Input: dimensioned drawing with shaded views. Units: mm. Origin: part minimum x, y, z. Give positions to 0.01 mm unless a question says otherwise; leave off trailing zeros. Loops run counter-clockwise (first coordinate to the right, second up) from the corner with the lowest first, then second, coordinate; pieces in that order, holes last. Notation, with made-up numbers: M 54,-4 L 103,-4 A14 cw 103,6 Z; hole C 44.5,-26 d1. An arc over 180 degrees is marked long. Use CSV: the item, a comma, the result in double quotes. Start each with the question number.
Q1. Pin query (flat end, axial travel): pin 1 (2 mm diameter, centred on x = 2.5, z = 53.5, fed in from -Y) (1 decimal); pin 2 (1 mm diameter, centred on x = 3, y = 63, fed in from +Z); pin 3 (1.5 mm diameter, centred on x = 1, y = 137, fed in from -Z). Return the tip coordinate at first contact, or that it passes through.
Q2. Section A-A, the plane x = 1.5. Output: boundary loops of the cut face in (y, z) (1 decimal), plus the area to 3 significant figures.
Q3. Section C-C, the plane z = 10. Output: boundary loops of the cut face in (x, y).
Q4. Material intervals for line 1 along Y through (x, z) = (4.75, 50) (1 decimal); line 2 along Z through (x, y) = (4, 18) (1 decimal); line 3 along Z through (x, y) = (1.5, 126), sorted ascending.
Q5. Section B-B, the plane y = 112. Output: boundary loops of the cut face in (x, z).
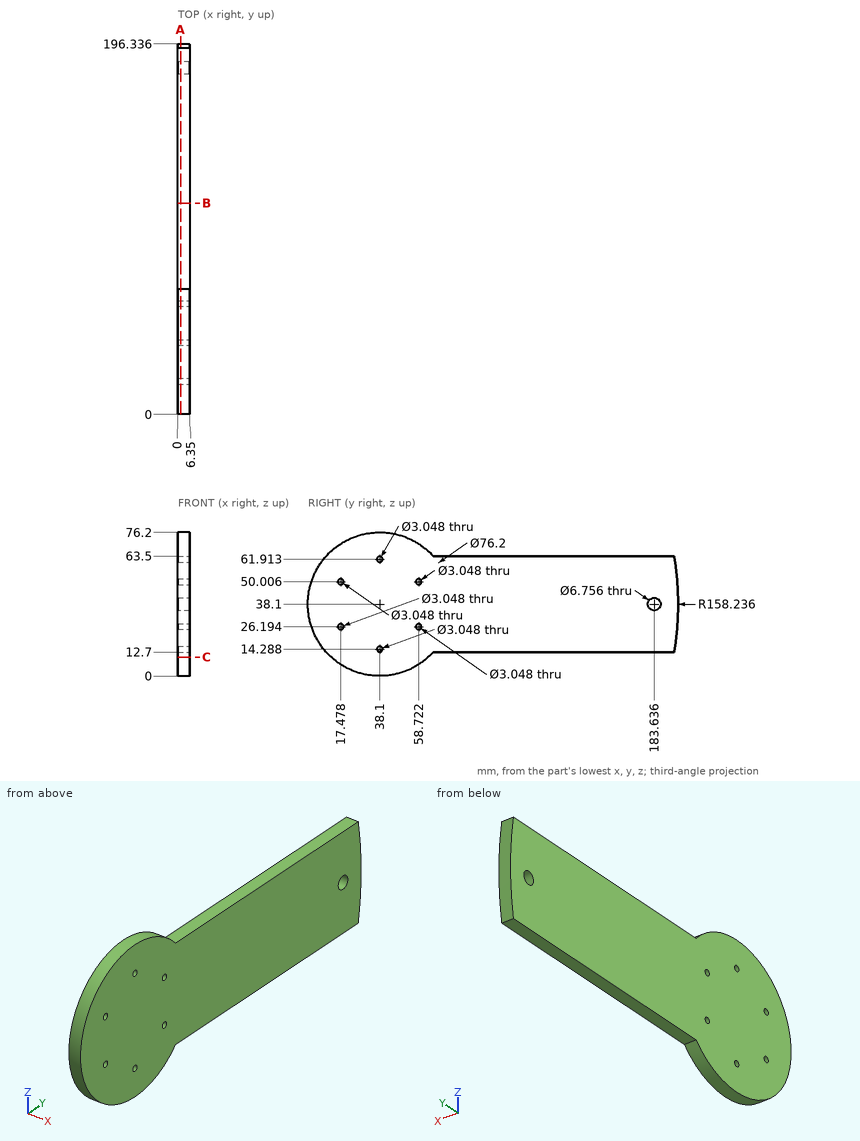
A:
1,pin 1,"y = 2.8"
1,pin 2,"z = 67.36"
1,pin 3,"z = 12.7"
2,outline,"M 66.5,12.7 L 194.3,12.7 A158.2 ccw 194.3,63.5 L 66.5,63.5 A38.1 ccw long Z; hole C 17.5,26.2 d3; hole C 17.5,50 d3; hole C 38.1,14.3 d3; hole C 38.1,61.9 d3; hole C 58.7,26.2 d3; hole C 58.7,50 d3; hole C 183.6,38.1 d6.8"
2,area,"10,700 mm^2"
3,outline,"M 0,12.37 L 6.35,12.37 L 6.35,63.83 L 0,63.83 Z"
4,line 1,"1.9 to 16, 19 to 57.2, 60.2 to 195.9"
4,line 2,"5.7 to 24.8, 27.6 to 48.6, 51.4 to 70.5"
4,line 3,"12.7 to 63.5"
5,outline,"M 0,12.7 L 6.35,12.7 L 6.35,63.5 L 0,63.5 Z"
